```python
from build123d import *

# Parameters (mm, degrees)
SKETCH1_R           = 2.75
BOSS_EXTRUDE1_DEPTH = 5
SKETCH2_R           = 4.5
BOSS_EXTRUDE2_DEPTH = 15
SKETCH3_W           = 30
SKETCH3_H           = 9
BOSS_EXTRUDE3_DEPTH = 30
SKETCH4_W           = 26
SKETCH4_H           = 7
CUT_EXTRUDE1_DEPTH  = 25
CUT_EXTRUDE2_DEPTH  = 39


with BuildPart() as part:
    # Sketch1 → Boss-Extrude1 (new body)
    with BuildSketch(Plane(origin=(0, 0, 0), x_dir=(1, 0, 0), z_dir=(0, 1, 0))):
        Circle(SKETCH1_R)
    extrude(amount=BOSS_EXTRUDE1_DEPTH)

    # Sketch2 → Boss-Extrude2 (add)
    with BuildSketch(Plane(origin=(0, 5, 0), x_dir=(1, 0, 0), z_dir=(0, 1, 0))):
        Circle(SKETCH2_R)
    extrude(amount=BOSS_EXTRUDE2_DEPTH)

    # Sketch3 → Boss-Extrude3 (add)
    with BuildSketch(Plane(origin=(0, 20, 0), x_dir=(1, 0, 0), z_dir=(0, 1, 0))):
        Rectangle(SKETCH3_W, SKETCH3_H)
    extrude(amount=BOSS_EXTRUDE3_DEPTH)

    # Sketch4 → Cut-Extrude1 (cut)
    with BuildSketch(Plane(origin=(0, 50, 0), x_dir=(1, 0, 0), z_dir=(0, 1, 0))):
        with Locations((0, 1)):
            Rectangle(SKETCH4_W, SKETCH4_H)
    extrude(amount=-CUT_EXTRUDE1_DEPTH, mode=Mode.SUBTRACT)

    # Sketch5 → Cut-Extrude2 (cut)
    with BuildSketch(Plane(origin=(15, 0, 0), x_dir=(0, 0, -1), z_dir=(1, 0, 0))):
        Polygon((-2.5, 50), (4.5, 25), (4.5, 50), align=None)
    extrude(amount=-CUT_EXTRUDE2_DEPTH, mode=Mode.SUBTRACT)


solid = part.part
```
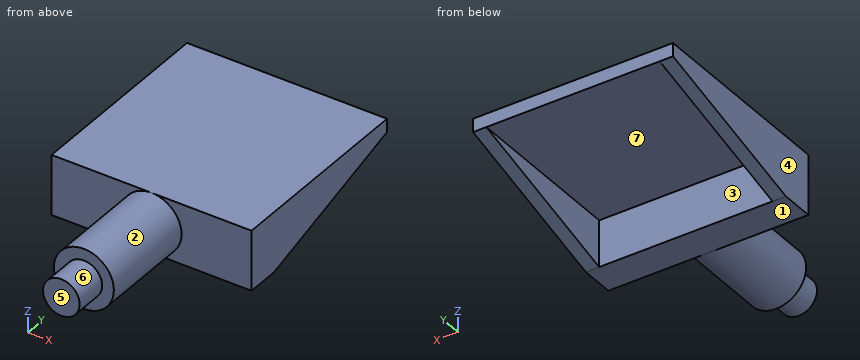
Can you work these out from the model? Positions are in its coordinate system, mm. Face numbers are marked on the shaded views. A direction names the side the tool comes from. Coordinates: 2 decimals unless noted, no trailing zeros. Loops run counter-clockwise (first coordinate to the right, second up) from the corner with the lowest first, then second, coordinate; pieces in that order, holes last. Notation, with made-up numbers: (-29, 30) - (-8, 30) arc R13 cw to (-8, 54) - close; hole circle Ø6 at (0, -14.5). An arc over 180 degrees is marked (long way). Answer as CSV lines item,"result". Start each with the question number.
1) Suppose I cut it at C-C (z = -1.75). Please give me the cut outline in (x, y).
2) Suppose I cut it at B-B (y = 35.5). Please give me the cut outline in (x, z).
3) Suppose I cut it at D-D (x = 3.5). Please give me the cut outline in (y, z).
4) Thinking about a two-plate mould opening in X: for the marked faces 1, 2, 3 and 4, which applies, pulls with the +X half, pulls with the -X half, needs draft (parallel to the pull), parting line crosses it, or undercut?
5) For pin 1 (4.5 mm diameter, centred on x = -7.5, z = -0.5, fed in from -Y); pin 2 (1 mm diameter, centred on x = 5.5, z = -2.5, fed in from +Y); pin 3 (2 mm diameter, centred on y = 37.5, z = -1.5, fed in from +X); pin 4 (5 mm diameter, centred on x = 1, y = 37, fed in from -Z), each with a flat end and sliding along its axis, tell me the tip position at first contact or that it passes through.
6) Suppose I cut it at A-A (x = 8.5). Please give me the cut outline in (y, z), plus the area to 3 significant figures.
7) Which directions (+Z, -Z, +X, -X, +Y, -Y) give clear straight access to the entire face, cutting with the end or side of a thin tool? Please do the marked faces 5, 6 and 7.
8) I need wall thicknesses on line 1 (X direction, y = 25.5, z = -3.75); line 2 (Y direction, x = -5, z = -0.75); line 3 (Z direction, x = 0, y = 36). Which ranges of each line are inside material? Lowest first, please. Write a range as from..to.
Check result:
1,outline,"(-15, 20) - (-4.15, 20) - (-4.15, 5) - (-2.12, 5) - (-2.12, 0) - (2.12, 0) - (2.12, 5) - (4.15, 5) - (4.15, 20) - (15, 20) - (15, 34.82) - (13, 34.82) - (13, 25) - (-13, 25) - (-13, 34.82) - (-15, 34.82) - close"
2,outline,"(-15, -1.56) - (-13, -1.56) - (-13, 2.5) - (13, 2.5) - (13, -1.56) - (15, -1.56) - (15, 4.5) - (-15, 4.5) - close"
3,outline,"(5, -2.83) - (20, -2.83) - (20, -4.5) - (25, -4.5) - (25, 2.5) - (50, 2.5) - (50, 4.5) - (20, 4.5) - (20, 2.83) - (5, 2.83) - close"
4,face 1,"needs draft"
4,face 2,"parting line crosses it"
4,face 3,"undercut"
4,face 4,"pulls with the -X half"
5,pin 1,"stops at y = 20"
5,pin 2,"stops at y = 25"
5,pin 3,"stops at x = 15"
5,pin 4,"stops at z = 2.5"
6,outline,"(20, -4.5) - (25, -4.5) - (25, 2.5) - (50, 2.5) - (50, 4.5) - (20, 4.5) - close"
6,area,"95.0 mm²"
7,face 5,"+Z, -Z, +X, -X, -Y"
7,face 6,"-Y"
7,face 7,"-Z, +Y"
8,line 1,"x = -15..-13, 13..15"
8,line 2,"y = 20..25"
8,line 3,"z = 2.5..4.5"
